The drawing under review shows one solid part. Ordinate dimensions are in mm from its lowest x, y, z. A direction names the side the tool comes from. Give positions to 0.01 mm unless a question says otherwise; leave off trailing zeros. Write each loop counter-clockwise with the first axis right and the second up, starting at its lowest first coordinate (ties: lowest second). Pieces come first, ordered by that corner, then holes.
Q1. We need section A-A (x = 7.25). Write out the cut boundary in (y, z), then the cut area to 3 significant figures.
Q2. We need section C-C (z = 27). Write out the cut boundary in (x, y).
Q3. For line 1 (Y direction, x = 2.35, z = 30); line 2 (Z direction, x = 14.75, y = 29.5); line 3 (Y direction, x = 4.5, z = 31) (3 decimals), list the stretches that pass through material, from the lowest coordinate up.
Q4. Machinability: for the marked faces 1 and 2, which of the approach directions +Z, -Z, +X, -X, +Y, -Y give a long, thin tool a straight path to every point of the face, cutting with its end or side? Answer none if there is none.
Q5. Insertion check: P1, Ø1, axis at x = 11, z = 42.5, coming from the +Y side; P2, Ø2, axis at x = 4.5, z = 31.5, coming from the -Y side; P3, Ø3, axis at x = 7, z = 7, coming from the -Y side; P4, Ø8, axis at x = 7, y = 9.5, coming from the +Z side. Each pin has a flat end and moves straight along its axis. Give the tip position at first contact, or say it passes through.
Q6. We need section D-D (y = 16). Write out the cut boundary in (x, z).
Q7. We need section B-B (y = 5). Write out the cut boundary in (x, z).
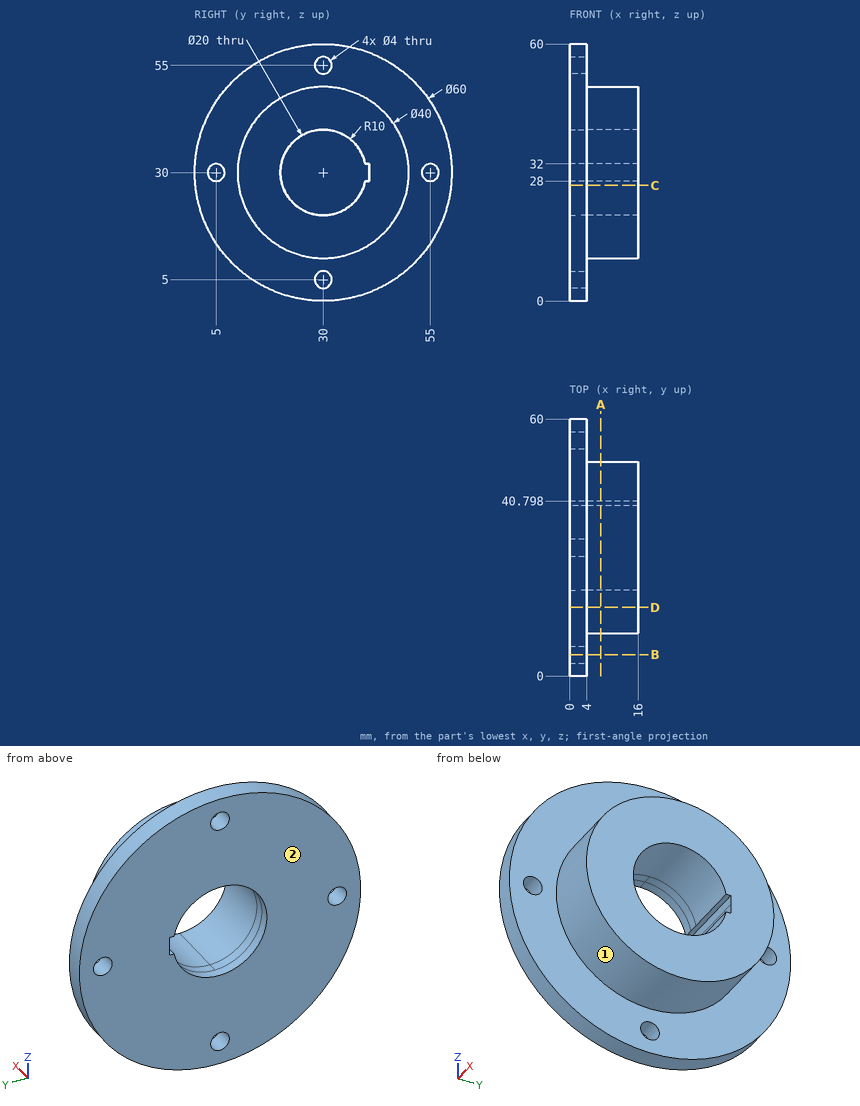
Computed:
1. outline: circle Ø40 at (30, 30); hole (39.8, 28) - (40.8, 28) - (40.8, 32) - (39.8, 32) arc R10 ccw (long way) to start
1. area: 939 mm2
2. outline: (0, 0.15) - (4, 0.15) - (4, 10.23) - (16, 10.23) - (16, 20.46) - (0, 20.46) - close; (0, 39.54) - (16, 39.54) - (16, 49.77) - (4, 49.77) - (4, 59.85) - (0, 59.85) - close
3. line 1: y = 0 to 3, 7 to 20, 40.8 to 53, 57 to 60
3. line 2: z = 10.01 to 20.01, 39.99 to 49.99
3. line 3: y = 10.025 to 20.05, 40.798 to 49.975
4. face 1: +X
4. face 2: +Z, -Z, -X, +Y, -Y
5. P1: stops at y = 46
5. P2: stops at y = 0.01
5. P3: passes through
5. P4: stops at z = 54.11
6. outline: (0, 3.47) - (4, 3.47) - (4, 15.72) - (16, 15.72) - (16, 44.28) - (4, 44.28) - (4, 56.53) - (0, 56.53) - close
7. outline: (0, 13.42) - (4, 13.42) - (4, 28) - (0, 28) - close; (0, 32) - (4, 32) - (4, 46.58) - (0, 46.58) - close
